Here's the drawing with two shaded views (mm, measured from the low corner). I have some questions. A direction names the side the tool comes from. Round coordinates to 2 decimals unless told otherwise and drop trailing zeros. Loops run counter-clockwise (first coordinate to the right, second up) from the corner with the lowest first, then second, coordinate; pieces in that order, holes last.
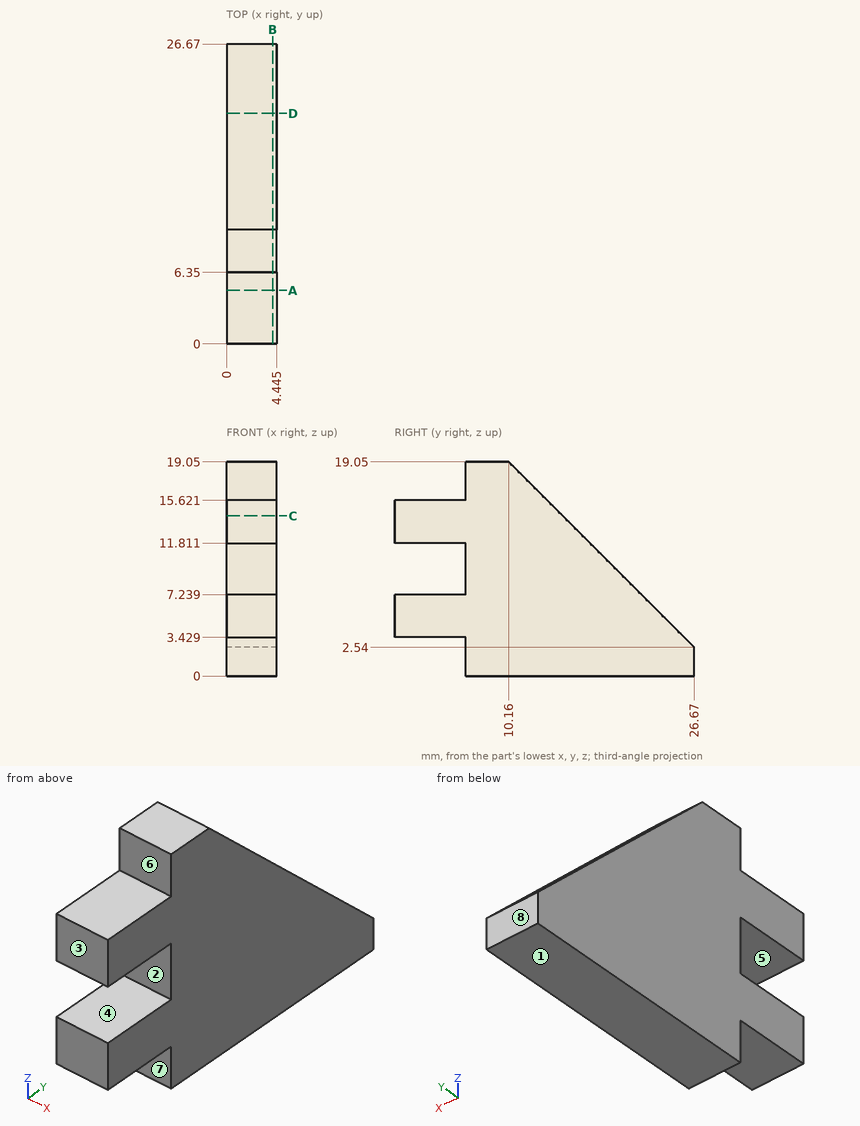
(1) If we section it at B-B, the plane x = 4.1: List the corners of the cut face in (y, z) for me.
Worked answers:
outline: (0, 3.43) - (6.35, 3.43) - (6.35, 0) - (26.67, 0) - (26.67, 2.54) - (10.16, 19.05) - (6.35, 19.05) - (6.35, 15.62) - (0, 15.62) - (0, 11.81) - (6.35, 11.81) - (6.35, 7.24) - (0, 7.24) - close
(2) If we section it at A-A, the plane y = 4.75: List the corners of the cut face in (x, z) for me (3 decimals), then the cut area to 3 significant figures.
Worked answers:
outline: (0, 3.429) - (4.445, 3.429) - (4.445, 7.239) - (0, 7.239) - close; (0, 11.811) - (4.445, 11.811) - (4.445, 15.621) - (0, 15.621) - close
area: 33.9 mm2
(3) For the marked faces 5, 6, 7 and 8, which set-ups out of +Z, -Z, +X, -X, +Y, -Y let a thin tool reach every point of the face, with its end or its side?
Worked answers:
face 5: +X, -X, -Y
face 6: +Z, +X, -X, -Y
face 7: -Z, +X, -X, -Y
face 8: +Z, -Z, +X, -X, +Y
(4) Will these pins go through, and if not, where does the flat tip stop? P1, Ø1.3, axis at x = 1, y = 3.5, coming from the -Z side; P2, Ø1, axis at x = 2.5, z = 13.5, coming from the +Y side; P3, Ø2, axis at x = 1.5, y = 3, coming from the +Z side.
Worked answers:
P1: stops at z = 3.43
P2: stops at y = 16.21
P3: stops at z = 15.62
(5) If we section it at D-D, the plane y = 20.5: List the corners of the cut face in (x, z) for me (3 decimals), then the cut area to 3 significant figures.
Worked answers:
outline: (0, 0) - (4.445, 0) - (4.445, 8.71) - (0, 8.71) - close
area: 38.7 mm2
(6) If we mould it in two halves opening along Z, with no side actions, what happens to the marked faces 1, 2, 3 and 4? For each: released by +Z, released by -Z, zero draft, split by the parting line, or undercut.
Worked answers:
face 1: released by -Z
face 2: undercut
face 3: zero draft
face 4: undercut
(7) If we section it at C-C, the plane z = 14.25: List the corners of the cut face in (x, y) for me (3 decimals), then the cut area to 3 significant figures.
Worked answers:
outline: (0, 0) - (4.445, 0) - (4.445, 14.96) - (0, 14.96) - close
area: 66.5 mm2
(8) If I drill on line 1 (Z direction, x = 1.25, y = 15); line 2 (Y direction, x = 3.45, z = 3); line 3 (Z direction, x = 3.9, y = 21.25), over which ranges is the centre line in solid material (lowest first)?
Worked answers:
line 1: z = 0 to 14.21
line 2: y = 6.35 to 26.21
line 3: z = 0 to 7.96
